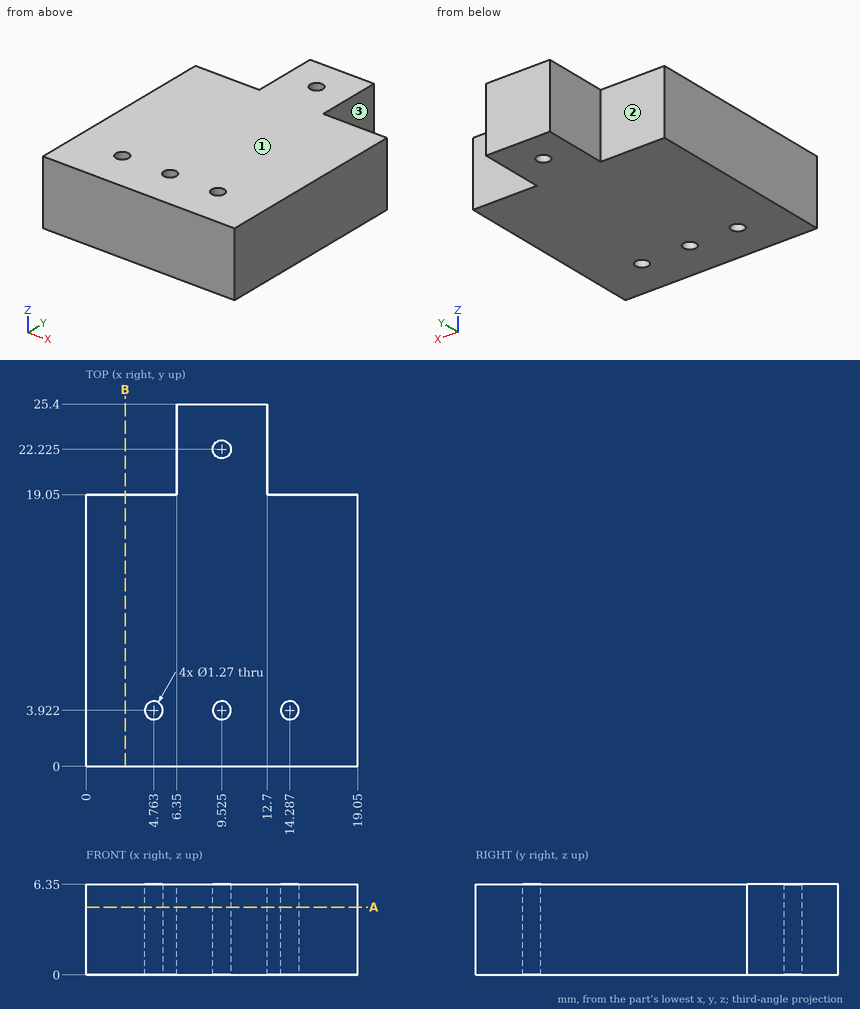
Print and shaded views of the part. All mm, measured from the part's lowest x, y and z. A direction names the side the tool comes from. Round coordinates to 2 decimals unless told otherwise and drop trailing zeros. Order: outer loops, then holes, each group sorted by start corner. A loop starts at its lowest first (then second) coordinate and runs counter-clockwise, first axis right, second up. Notation, with made-up numbers: (-34, 0.5) - (-26, 0.5) arc R19 cw to (-26, 6.5) - close; hole circle Ø2 at (-28.75, 69). An arc over 180 degrees is marked (long way). Use a Markdown table: item, result.
1) Tool access for the marked faces 1, 2 and 3: list every direction of +Z, -Z, +X, -X, +Y, -Y with a clear straight run to the whole face (end or side of a thin tool).
Recorded:
| item | result |
|---|---|
| face 1 | +Z, +X, -X, +Y, -Y |
| face 2 | +Z, -Z, -X, +Y |
| face 3 | +Z, -Z, +X, +Y |
2) Saw through at A-A on z = 4.75. Give the number of separate pieces and of enclosed holes in the cut face, and give its area (3 significant figures).
Recorded:
| item | result |
|---|---|
| separate pieces | 1 |
| enclosed holes | 4 |
| area | 398 mm² |
3) Wall check: L1, parallel to Y at x = 9.5, z = 3.5; L2, parallel to Y at x = 3.5, z = 2; L3, parallel to X at y = 23, z = 2. Give the ranges that are in metal, low to high.
Recorded:
| item | result |
|---|---|
| L1 | y = 0 to 3.29, 4.56 to 21.59, 22.86 to 25.4 |
| L2 | y = 0 to 19.05 |
| L3 | x = 6.35 to 12.7 |
4) Saw through at B-B on x = 2.75. Write the cut outline in (y, z), and give its area (3 significant figures).
Recorded:
| item | result |
|---|---|
| outline | (0, 0) - (19.05, 0) - (19.05, 6.35) - (0, 6.35) - close |
| area | 121 mm² |
5) Flat gauge pins, fed straight in: pin 1 Ø1.1 at (x, y) = (14.29, 3.92) entering from -Z; pin 2 Ø2 at (x, z) = (16, 2.5) entering from +Y; pin 3 Ø2 at (y, z) = (20.5, 4.5) entering from -X; pin 4 Ø1.9 at (y, z) = (21.5, 2.5) entering from +X. Where does each tip first touch, or does it go through?
Recorded:
| item | result |
|---|---|
| pin 1 | passes through |
| pin 2 | stops at y = 19.05 |
| pin 3 | stops at x = 6.35 |
| pin 4 | stops at x = 12.7 |
